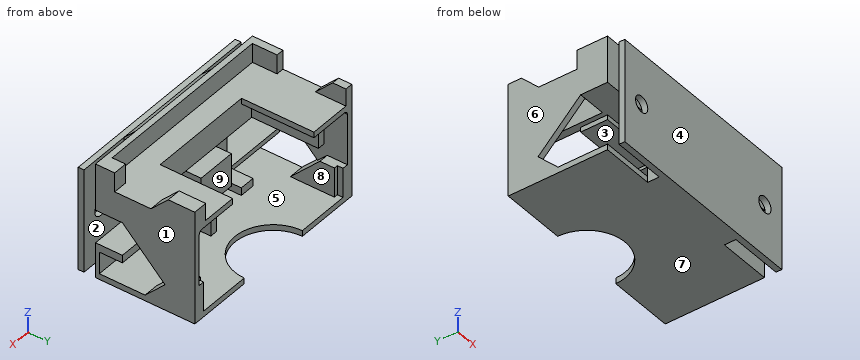
```python
from build123d import *

# Parameters (mm, degrees)
SKETCH1_W                      = 54
SKETCH1_H                      = 27
BOSS_EXTRUDE1_DEPTH            = 1.5
CUT_EXTRUDE1_REACH             = 62.392
SKETCH2_R                      = 2.1
CUT_EXTRUDE1_DIRECTION_2_DEPTH = 61.392466418
SKETCH3_W                      = 26.4
SKETCH3_H                      = 30
BOSS_EXTRUDE2_DEPTH            = 3
CHAMFER3_SIZE                  = 3
BOSS_EXTRUDE3_DEPTH            = 7
BOSS_EXTRUDE15_START           = 7
SKETCH4_4_W                    = 10.4
SKETCH4_4_H                    = 8.6
BOSS_EXTRUDE15_DEPTH           = 4
SKETCH5_W                      = 54
SKETCH5_H                      = 1.5
BOSS_EXTRUDE5_DEPTH            = 18.86
SKETCH5_3_W                    = 2
SKETCH5_3_H                    = 5.7
BOSS_EXTRUDE6_DEPTH            = 17.36
SKETCH4_3_W                    = 8
SKETCH4_3_H                    = 8.6
BOSS_EXTRUDE12_DEPTH           = 3.86
SKETCH17_W                     = 2
SKETCH17_H                     = 6.43
SKETCH17_W_2                   = 3.74
SKETCH17_H_2                   = 3.5
BOSS_EXTRUDE13_DEPTH           = 5
SKETCH17_3_W                   = 2
SKETCH17_3_H                   = 7.93
SKETCH17_3_W_2                 = 3.74
SKETCH17_3_H_2                 = 11.43
BOSS_EXTRUDE16_DEPTH           = 4.5
CHAMFER7_SIZE                  = 4.5
SKETCH5_4_W                    = 54
SKETCH5_4_H                    = 1.5
BOSS_EXTRUDE8_DEPTH            = 18.86
BOSS_EXTRUDE9_DEPTH            = 1.5
SKETCH18_W                     = 4
SKETCH18_H                     = 7.7
BOSS_EXTRUDE14_DEPTH           = 13
CHAMFER6_SIZE                  = 7.75
SKETCH20_W                     = 1
SKETCH20_H                     = 7.7
CUT_EXTRUDE7_DEPTH             = 1.5
SKETCH12_W                     = 28
SKETCH12_H                     = 18.86
CUT_EXTRUDE2_DEPTH             = 7.2
SKETCH14_R                     = 10
CUT_EXTRUDE3_DEPTH             = 10
SKETCH15_W                     = 4
SKETCH15_H                     = 2
BOSS_EXTRUDE11_DEPTH           = 6
SKETCH21_W                     = 17
SKETCH21_H                     = 5.7
SKETCH21_H_2                   = 0.75
CUT_EXTRUDE8_DEPTH             = 6
CUT_EXTRUDE9_START             = -6
SKETCH21_3_W                   = 17
SKETCH21_3_H                   = 5.7
SKETCH21_3_H_2                 = 0.75
CUT_EXTRUDE9_DEPTH             = 1
FILLET7_R                      = 1


# Some blends are built 0.0001 mm under size
with BuildPart() as part:
    # Sketch1 → Boss-Extrude1 (new body)
    with BuildSketch(Plane(origin=(0, 0, 0), x_dir=(1, 0, 0), z_dir=(0, 1, 0))):
        with Locations((27, 13.5)):
            Rectangle(SKETCH1_W, SKETCH1_H)
    extrude(amount=BOSS_EXTRUDE1_DEPTH)

    # Sketch2 → Cut-Extrude1 (cut, up to next)
    with BuildSketch(Plane(origin=(0, 1.5, 0), x_dir=(1, 0, 0), z_dir=(0, 1, 0)), mode=Mode.PRIVATE) as cut_extrude1_sk1:
        with Locations(Location((5.8, 13.5, 0), (0, 0, 90))):
            Circle(SKETCH2_R)
    cut_extrude1_tool1 = extrude(cut_extrude1_sk1.sketch, amount=-CUT_EXTRUDE1_REACH, mode=Mode.PRIVATE) & part.part
    cut_extrude1 = cut_extrude1_tool1.solids().sort_by_distance((5.8, 1.5, -13.5))[0]
    add(cut_extrude1, mode=Mode.SUBTRACT)

    # Sketch2 → Cut-Extrude1 direction 2 (cut)
    with BuildSketch(Plane(origin=(0, 1.5, 0), x_dir=(1, 0, 0), z_dir=(0, 1, 0))):
        with Locations(Location((5.8, 13.5, 0), (0, 0, 90))):
            Circle(SKETCH2_R)
    cut_extrude1_direction_2 = extrude(amount=CUT_EXTRUDE1_DIRECTION_2_DEPTH, mode=Mode.SUBTRACT)

    # Mirror1: Cut-Extrude1, Cut-Extrude1 direction 2 across plane
    add(cut_extrude1.mirror(Plane.ZY.offset(-27)), mode=Mode.SUBTRACT)
    add(cut_extrude1_direction_2.mirror(Plane.ZY.offset(-27)), mode=Mode.SUBTRACT)

    # Sketch3 → Boss-Extrude2 (add)
    with BuildSketch(Plane(origin=(0, 1.5, 0), x_dir=(1, 0, 0), z_dir=(0, 1, 0))):
        with Locations((27, 12)):
            Rectangle(SKETCH3_W, SKETCH3_H)
    extrude(amount=BOSS_EXTRUDE2_DEPTH)

    # Chamfer3
    chamfer3_edges = [part.edges().sort_by_distance(p)[0] for p in [
        (27, 1.5, 3),
    ]]
    chamfer(chamfer3_edges, length=CHAMFER3_SIZE - 0.0001)  # a hair under: the kernel refuses the full size

    # Sketch4 → Boss-Extrude3 (add)
    with BuildSketch(Plane(origin=(0, 4.5, 0), x_dir=(1, 0, 0), z_dir=(0, 1, 0))):
        Polygon((54, 27), (0, 27), (0, 17.8), (21.8, 17.8), (21.8, 9.2), (0, 9.2), (0, 2), (54, 2), (54, 9.2), (32.2, 9.2), (32.2, 17.8), (54, 17.8), align=None)
    extrude(amount=BOSS_EXTRUDE3_DEPTH)

    # Sketch4<4> → Boss-Extrude15 (add)
    with BuildSketch(Plane(origin=(0, 4.5, 0), x_dir=(1, 0, 0), z_dir=(0, 1, 0)).offset(BOSS_EXTRUDE15_START)):
        with Locations((27, 13.5)):
            Rectangle(SKETCH4_4_W, SKETCH4_4_H)
    extrude(amount=BOSS_EXTRUDE15_DEPTH)

    # Sketch5 → Boss-Extrude5 (add)
    with BuildSketch(Plane(origin=(0, 11.5, 0), x_dir=(1, 0, 0), z_dir=(0, 1, 0))):
        with Locations((27, 2.75)):
            Rectangle(SKETCH5_W, SKETCH5_H)
    extrude(amount=BOSS_EXTRUDE5_DEPTH)

    # Sketch5<3> → Boss-Extrude6 (add)
    with BuildSketch(Plane(origin=(0, 11.5, 0), x_dir=(1, 0, 0), z_dir=(0, 1, 0))):
        with Locations((45.5, 6.35)):
            Rectangle(SKETCH5_3_W, SKETCH5_3_H)
        with Locations((8.5, 6.35)):
            Rectangle(SKETCH5_3_W, SKETCH5_3_H)
    extrude(amount=BOSS_EXTRUDE6_DEPTH)

    # Sketch4<3> → Boss-Extrude12 (add)
    with BuildSketch(Plane(origin=(0, 4.5, 0), x_dir=(1, 0, 0), z_dir=(0, 1, 0))):
        with Locations((17.8, 13.5)):
            Rectangle(SKETCH4_3_W, SKETCH4_3_H)
        with Locations((36.2, 13.5)):
            Rectangle(SKETCH4_3_W, SKETCH4_3_H)
    extrude(amount=BOSS_EXTRUDE12_DEPTH)

    # Sketch17 → Boss-Extrude13 (add)
    with BuildSketch(Plane.XY.offset(-2)):
        with Locations((1, 9.215)):
            Rectangle(SKETCH17_W, SKETCH17_H)
        Polygon((0, 6), (0, 4.5), (13.8, 4.5), (40.2, 4.5), (54, 4.5), (54, 6), (50.26, 6), (2, 6), align=None)
        with Locations((52.13, 7.75)):
            Rectangle(SKETCH17_W_2, SKETCH17_H_2)
    extrude(amount=BOSS_EXTRUDE13_DEPTH)

    # Sketch17<3> → Boss-Extrude16 (add)
    with BuildSketch(Plane.XY.offset(-2)):
        with Locations((1, 26.395)):
            Rectangle(SKETCH17_3_W, SKETCH17_3_H)
        with Locations((52.13, 24.645)):
            Rectangle(SKETCH17_3_W_2, SKETCH17_3_H_2)
    extrude(amount=BOSS_EXTRUDE16_DEPTH)

    # Chamfer7
    chamfer7_edges = [part.edges().sort_by_distance(p)[0] for p in [
        (52.13, 18.93, 2.5),
        (1, 22.43, 2.5),
    ]]
    chamfer(chamfer7_edges, length=CHAMFER7_SIZE - 0.0001)  # a hair under: the kernel refuses the full size

    # Sketch5<4> → Boss-Extrude8 (add)
    with BuildSketch(Plane(origin=(0, 11.5, 0), x_dir=(1, 0, 0), z_dir=(0, 1, 0))):
        with Locations((27, 26.25)):
            Rectangle(SKETCH5_4_W, SKETCH5_4_H)
    extrude(amount=BOSS_EXTRUDE8_DEPTH)

    # Sketch10 → Boss-Extrude9 (add)
    with BuildSketch(Plane.ZY):
        Polygon((-3.5, 11.5), (-3.5, 30.36), (-25.5, 30.36), (-25.5, 27.8), (-9.2, 11.5), align=None)
    boss_extrude9 = extrude(amount=-BOSS_EXTRUDE9_DEPTH)

    # Mirror3: Boss-Extrude9 across plane
    add(boss_extrude9.mirror(Plane.ZY.offset(-27)))

    # Sketch18 → Boss-Extrude14 (add)
    with BuildSketch(Plane(origin=(0, 30.36, 0), x_dir=(1, 0, 0), z_dir=(0, 1, 0))):
        with Locations((2, 21.65)):
            Rectangle(SKETCH18_W, SKETCH18_H)
        with Locations((52, 21.65)):
            Rectangle(SKETCH18_W, SKETCH18_H)
    extrude(amount=-BOSS_EXTRUDE14_DEPTH)

    # Chamfer6
    # the kernel refuses this chamfer: 7.75 mm, written as the material it takes off along each edge
    with BuildSketch(Plane(origin=(23.930543157, 17.36, -17.8), x_dir=(0, -0.027495876610586188, -0.9996219169112968), z_dir=(-1, 0, 0))) as chamfer6_piece_1_section:
        Polygon((CHAMFER6_SIZE * 0.999621916911, -CHAMFER6_SIZE * 0.0274958766106), (-CHAMFER6_SIZE * 0.0274958766106, -CHAMFER6_SIZE * 0.999621916911), (0, 0), align=None)
    chamfer6_piece_1 = extrude(amount=43.861086313, mode=Mode.PRIVATE)
    chamfer6_piece_1 = split(chamfer6_piece_1, bisect_by=Plane(origin=(2.75, 21.192634452, -18.892634452), z_dir=(0, -0.7071067811865515, -0.7071067811865436)), keep=Keep.TOP, mode=Mode.PRIVATE)
    chamfer6_piece_1 = split(chamfer6_piece_1, bisect_by=Plane(origin=(2.75, 19.24037252, -25.5), z_dir=(0, 0, 1)), keep=Keep.TOP, mode=Mode.PRIVATE)
    add(chamfer6_piece_1, mode=Mode.SUBTRACT)
    with BuildSketch(Plane(origin=(23.930543157, 17.36, -17.8), x_dir=(0, -0.027495876610586188, -0.9996219169112968), z_dir=(-1, 0, 0))) as chamfer6_piece_2_section:
        Polygon((CHAMFER6_SIZE * 0.999621916911, -CHAMFER6_SIZE * 0.0274958766106), (-CHAMFER6_SIZE * 0.0274958766106, -CHAMFER6_SIZE * 0.999621916911), (0, 0), align=None)
    chamfer6_piece_2 = extrude(amount=43.861086313, mode=Mode.PRIVATE)
    chamfer6_piece_2 = split(chamfer6_piece_2, bisect_by=Plane(origin=(1.5, 22.605, -18.635), z_dir=(1, 0, 0)), keep=Keep.TOP, mode=Mode.PRIVATE)
    chamfer6_piece_2 = split(chamfer6_piece_2, bisect_by=Plane(origin=(2.75, 22.605, -25.5), z_dir=(0, 0, 1)), keep=Keep.TOP, mode=Mode.PRIVATE)
    add(chamfer6_piece_2, mode=Mode.SUBTRACT)
    with BuildSketch(Plane(origin=(73.930543157, 17.36, -17.8), x_dir=(0, 0.9996219169112968, 0.027495876610586188), z_dir=(-1, 0, 0))) as chamfer6_piece_3_section:
        Polygon((CHAMFER6_SIZE * 0.999621916911, CHAMFER6_SIZE * 0.0274958766106), (-CHAMFER6_SIZE * 0.0274958766106, CHAMFER6_SIZE * 0.999621916911), (0, 0), align=None)
    chamfer6_piece_3 = extrude(amount=43.861086313, mode=Mode.PRIVATE)
    chamfer6_piece_3 = split(chamfer6_piece_3, bisect_by=Plane(origin=(53.25, 21.192634452, -18.892634452), z_dir=(0, -0.7071067811865515, -0.7071067811865436)), keep=Keep.TOP, mode=Mode.PRIVATE)
    chamfer6_piece_3 = split(chamfer6_piece_3, bisect_by=Plane(origin=(53.25, 19.24037252, -25.5), z_dir=(0, 0, 1)), keep=Keep.TOP, mode=Mode.PRIVATE)
    add(chamfer6_piece_3, mode=Mode.SUBTRACT)
    with BuildSketch(Plane(origin=(73.930543157, 17.36, -17.8), x_dir=(0, 0.9996219169112968, 0.027495876610586188), z_dir=(-1, 0, 0))) as chamfer6_piece_4_section:
        Polygon((CHAMFER6_SIZE * 0.999621916911, CHAMFER6_SIZE * 0.0274958766106), (-CHAMFER6_SIZE * 0.0274958766106, CHAMFER6_SIZE * 0.999621916911), (0, 0), align=None)
    chamfer6_piece_4 = extrude(amount=43.861086313, mode=Mode.PRIVATE)
    chamfer6_piece_4 = split(chamfer6_piece_4, bisect_by=Plane(origin=(52.5, 22.605, -18.635), z_dir=(-1, 0, 0)), keep=Keep.TOP, mode=Mode.PRIVATE)
    chamfer6_piece_4 = split(chamfer6_piece_4, bisect_by=Plane(origin=(51.25, 22.605, -25.5), z_dir=(0, 0, 1)), keep=Keep.TOP, mode=Mode.PRIVATE)
    add(chamfer6_piece_4, mode=Mode.SUBTRACT)

    # Sketch20 → Cut-Extrude7 (cut)
    with BuildSketch(Plane(origin=(0, 30.36, 0), x_dir=(1, 0, 0), z_dir=(0, 1, 0))):
        with Locations((3.5, 21.65)):
            Rectangle(SKETCH20_W, SKETCH20_H)
        with Locations((50.5, 21.65)):
            Rectangle(SKETCH20_W, SKETCH20_H)
    extrude(amount=-CUT_EXTRUDE7_DEPTH, mode=Mode.SUBTRACT)

    # Sketch12 → Cut-Extrude2 (cut)
    with BuildSketch(Plane.XY.offset(-2)):
        with Locations((27, 20.93)):
            Rectangle(SKETCH12_W, SKETCH12_H)
    extrude(amount=-CUT_EXTRUDE2_DEPTH, mode=Mode.SUBTRACT)

    # Sketch14 → Cut-Extrude3 (cut)
    with BuildSketch(Plane(origin=(0, 0, -27), x_dir=(-1, 0, 0), z_dir=(0, 0, -1))):
        with Locations((-27, 30.36)):
            Circle(SKETCH14_R)
    extrude(amount=-CUT_EXTRUDE3_DEPTH, mode=Mode.SUBTRACT)

    # Sketch15 → Boss-Extrude11 (add)
    with BuildSketch(Plane(origin=(0, 11.5, 0), x_dir=(1, 0, 0), z_dir=(0, 1, 0))):
        with Locations((19, 18.8)):
            Rectangle(SKETCH15_W, SKETCH15_H)
    boss_extrude11 = extrude(amount=BOSS_EXTRUDE11_DEPTH)

    # Mirror5: Boss-Extrude11 across plane
    add(boss_extrude11.mirror(Plane.ZY.offset(-27)))

    # Sketch21 → Cut-Extrude8 (cut)
    with BuildSketch(Plane(origin=(0, 11.5, 0), x_dir=(1, 0, 0), z_dir=(0, 1, 0))):
        Polygon((54, 25.5), (17, 25.5), (17, 19.8), (21, 19.8), (33, 19.8), (37, 19.8), (54, 19.8), align=None)
        with Locations((8.5, 22.65)):
            Rectangle(SKETCH21_W, SKETCH21_H)
        with Locations((8.5, 19.425)):
            Rectangle(SKETCH21_W, SKETCH21_H_2)
    extrude(amount=-CUT_EXTRUDE8_DEPTH, mode=Mode.SUBTRACT)

    # Sketch21<3> → Cut-Extrude9 (cut)
    with BuildSketch(Plane(origin=(0, 11.5, 0), x_dir=(1, 0, 0), z_dir=(0, 1, 0)).offset(CUT_EXTRUDE9_START)):
        with Locations((8.5, 22.65)):
            Rectangle(SKETCH21_3_W, SKETCH21_3_H)
        with Locations((8.5, 19.425)):
            Rectangle(SKETCH21_3_W, SKETCH21_3_H_2)
    extrude(amount=-CUT_EXTRUDE9_DEPTH, mode=Mode.SUBTRACT)

    # Fillet7
    fillet7_edges = [part.edges().sort_by_distance(p)[0] for p in [
        (1.5, 20.93, -3.5),
        (52.5, 20.93, -3.5),
    ]]
    fillet(fillet7_edges, radius=FILLET7_R)


solid = part.part
```
Work out the finished part from the listing and answer in its coordinate system (mm). Face numbers are marked on the shaded views. A direction names the side the tool comes from. Give positions to 0.01 mm unless a question says otherwise; leave off trailing zeros. Loops run counter-clockwise (first coordinate to the right, second up) from the corner with the lowest first, then second, coordinate; pieces in that order, holes last. Notation, with made-up numbers: M -38.75,71.25 L 2.25,71.25 A32 ccw 2.25,100.25 Z; hole C 49,-11.75 d10. An arc over 180 degrees is marked long. One line per item, written item: value. Start each with the question number.
1. Determine the mould class of the marked faces 1, 2, 3 and 4 for opening direction Y: released by +Y, released by -Y, zero draft, split by the parting line, or undercut.
2. Find section D-D (x = 5.8). Give the vertices of the cut face in (y, z).
3. Find section B-B (z = -24). Give the vertices of the cut face in (x, y).
4. Which of the six approach directions +Z, -Z, +X, -X, +Y, -Y give full straight-line access (tool end or side, diameter ignored) to the marked faces 5, 6, 7, 8 and 9?
5. Find section A-A (x = 48.2). Give the vertices of the cut face in (y, z), and give its area (3 significant figures).
6. Each of these flat-tipped pins is pushed along its axis until it touches: P1, Ø1, axis at x = 8.5, y = 22, coming from the +Z side; P2, Ø3, axis at x = 52, y = 25.5, coming from the +Z side; P3, Ø0.8, axis at x = 50.5, z = -20, coming from the +Y side; P4, Ø2.5, axis at y = 13.5, z = -22, coming from the -X side. Where does it stop, or does it pass through?
7. Find the intervals of material crossed by probe 1 along X at (y, z) = (1.15, -13.5); probe 2 along Z at (x, y) = (50, 12.5); probe 3 along X at (y, z) = (29.5, -11.5), in increasing order.
8. Find section C-C (z = -13.5). Give the vertices of the cut face in (x, y).
Reported:
1. face 1: zero draft
1. face 2: undercut
1. face 3: undercut
1. face 4: released by -Y
2. outline: M 0,-27 L 1.5,-27 L 1.5,-15.6 L 0,-15.6 Z; M 0,-11.4 L 1.5,-11.4 L 1.5,0 L 0,0 Z; M 4.5,-27 L 30.36,-27 L 30.36,-25.5 L 4.5,-25.5 Z; M 4.5,-19.05 L 11.5,-19.05 L 11.5,-17.8 L 4.5,-17.8 Z; M 4.5,-9.2 L 11.5,-9.2 L 11.5,-3.5 L 30.36,-3.5 L 30.36,-2 L 6,-2 L 6,3 L 4.5,3 Z
3. outline: M 0,0 L 54,0 L 54,1.5 L 40.2,1.5 L 40.2,4.5 L 54,4.5 L 54,5.5 L 17,5.5 L 17,4.5 L 13.8,4.5 L 13.8,1.5 L 0,1.5 Z; M 0,18.91 L 4,18.91 L 4,28.86 L 3,28.86 L 3,30.36 L 0,30.36 Z; M 50,18.91 L 54,18.91 L 54,30.36 L 51,30.36 L 51,28.86 L 50,28.86 Z
4. face 5: none
4. face 6: +Z, -Z, -X, +Y, -Y
4. face 7: -Z, +X, -X, +Y, -Y
4. face 8: +Y
4. face 9: +Z, +Y
5. outline: M 0,-27 L 1.5,-27 L 1.5,-15.6 L 0,-15.6 Z; M 0,-11.4 L 1.5,-11.4 L 1.5,0 L 0,0 Z; M 4.5,-27 L 30.36,-27 L 30.36,-25.5 L 5.5,-25.5 L 5.5,-19.8 L 11.5,-19.8 L 11.5,-17.8 L 4.5,-17.8 Z; M 4.5,-9.2 L 11.5,-9.2 L 11.5,-3.5 L 30.36,-3.5 L 30.36,-2 L 6,-2 L 6,3 L 4.5,3 Z
5. area: 179 mm²
6. P1: stops at z = -2
6. P2: stops at z = 2.5
6. P3: stops at y = 28.86
6. P4: passes through
7. probe 1: x = 0 to 3.7, 7.9 to 46.1, 50.3 to 54
7. probe 2: z = -27 to -25.5, -3.5 to -2
7. probe 3: x = 0 to 1.5, 52.5 to 54
8. outline: M 0,0 L 3.7,0 L 3.7,1.5 L 0,1.5 Z; M 0,15.8 L 1.5,15.8 L 1.5,30.36 L 0,30.36 Z; M 7.9,0 L 46.1,0 L 46.1,1.5 L 40.2,1.5 L 40.2,8.36 L 32.2,8.36 L 32.2,15.5 L 21.8,15.5 L 21.8,8.36 L 13.8,8.36 L 13.8,1.5 L 7.9,1.5 Z; M 50.3,0 L 54,0 L 54,1.5 L 50.3,1.5 Z; M 52.5,15.8 L 54,15.8 L 54,30.36 L 52.5,30.36 Z
